Source: CAD feature listing. Evaluate the final solid. Frame: model axes, mm. A direction names the side the tool comes from. Give positions to 0.01 mm unless a question says otherwise; leave off trailing zeros. Loops run counter-clockwise (first coordinate to the right, second up) from the corner with the lowest first, then second, coordinate; pieces in that order, holes last. Notation, with made-up numbers: M -5,12.5 L 2,12.5 A19 cw 2,22.5 Z; hole C -29,4 d4. An arc over 180 degrees is marked long. Put each result on its own line as item: value.
from build123d import *

# Parameters (mm, degrees)
SKETCH1_W           = 166
SKETCH1_H           = 96
BOSS_EXTRUDE1_DEPTH = 33
SKETCH2_W           = 150
SKETCH2_H           = 80
CUT_EXTRUDE1_DEPTH  = 30
BOSS_EXTRUDE2_DEPTH = 5
SKETCH5_W           = 75
SKETCH5_H           = 5
BOSS_EXTRUDE3_DEPTH = 5
LPATTERN1_COUNT     = 15
LPATTERN1_PITCH     = 10
CUT_EXTRUDE5_DEPTH  = 10
FILLET1_R           = 4
FILLET2_R           = 4
FILLET3_R           = 2
FILLET5_R           = 1
CHAMFER1_SIZE       = 0.5


with BuildPart() as part:
    # Sketch1 → Boss-Extrude1 (new body)
    with BuildSketch(Plane(origin=(0, 0, 0), x_dir=(1, 0, 0), z_dir=(0, 1, 0))):
        with Locations((18.075570249, -18.706715624)):
            Rectangle(SKETCH1_W, SKETCH1_H)
    extrude(amount=BOSS_EXTRUDE1_DEPTH)

    # Sketch2 → Cut-Extrude1 (cut)
    with BuildSketch(Plane(origin=(0, 33, 0), x_dir=(1, 0, 0), z_dir=(0, 1, 0))):
        with Locations((18.075570249, -18.706715624)):
            Rectangle(SKETCH2_W, SKETCH2_H)
    extrude(amount=-CUT_EXTRUDE1_DEPTH, mode=Mode.SUBTRACT)

    # Sketch4 → Boss-Extrude2 (add)
    with BuildSketch(Plane.ZY.offset(-93.075570249)):
        Polygon((53.706715624, 3), (-21.293284376, 8), (-21.293284376, 3), align=None)
    boss_extrude2 = extrude(amount=BOSS_EXTRUDE2_DEPTH)

    # Sketch5 → Boss-Extrude3 (add)
    with BuildSketch(Plane.ZY.offset(-88.075570249)):
        with Locations((16.206715624, 5.5)):
            Rectangle(SKETCH5_W, SKETCH5_H)
    boss_extrude3 = extrude(amount=BOSS_EXTRUDE3_DEPTH)

    # LPattern1: Boss-Extrude2, Boss-Extrude3 ×15
    with Locations(*[(-i * LPATTERN1_PITCH, 0, 0) for i in range(1, LPATTERN1_COUNT)]):
        add(boss_extrude2)
        add(boss_extrude3)

    # Sketch9 → Cut-Extrude5 (cut)
    with BuildSketch(Plane(origin=(0, 33, 0), x_dir=(1, 0, 0), z_dir=(0, 1, 0))):
        Polygon((-62.174429751, 26.543284376), (98.325570249, 26.543284376), (98.325570249, -58.706715624), (95.325570249, -58.706715624), (95.325570249, 23.543284376), (-59.174429751, 23.543284376), (-59.174429751, -58.706715624), (-62.174429751, -58.706715624), align=None)
    extrude(amount=-CUT_EXTRUDE5_DEPTH, mode=Mode.SUBTRACT)

    # Fillet1
    fillet1_edges = [part.edges().sort_by_distance(p)[0] for p in [
        (-64.924429751, 16.5, -29.293284376),
        (101.075570249, 16.5, -29.293284376),
        (101.075570249, 16.5, 66.706715624),
        (-64.924429751, 16.5, 66.706715624),
    ]]
    fillet(fillet1_edges, radius=FILLET1_R)

    # Fillet2
    fillet2_edges = [part.edges().sort_by_distance(p)[0] for p in [
        (-56.924429751, 18, 58.706715624),
        (93.075570249, 18, 58.706715624),
        (93.075570249, 20.5, -21.293284376),
        (-56.924429751, 20.5, -21.293284376),
    ]]
    fillet(fillet2_edges, radius=FILLET2_R)

    # Fillet3
    fillet3_edges = [part.edges().sort_by_distance(p)[0] for p in [
        (75.575570249, 8, 53.706715624),
        (65.575570249, 8, 53.706715624),
        (55.575570249, 8, 53.706715624),
        (45.575570249, 8, 53.706715624),
        (35.575570249, 8, 53.706715624),
        (25.575570249, 8, 53.706715624),
        (15.575570249, 8, 53.706715624),
        (5.575570249, 8, 53.706715624),
        (-4.424429751, 8, 53.706715624),
        (-14.424429751, 8, 53.706715624),
        (-24.424429751, 8, 53.706715624),
        (-34.424429751, 8, 53.706715624),
        (-44.424429751, 8, 53.706715624),
        (-54.424429751, 8, 53.706715624),
        (85.575570249, 8, 53.706715624),
    ]]
    fillet(fillet3_edges, radius=FILLET3_R)

    # Fillet5
    fillet5_edges = [part.edges().sort_by_distance(p)[0] for p in [
        (-64.924429751, 33, 18.706715624),
        (18.075570249, 33, -29.293284376),
        (18.075570249, 33, 66.706715624),
        (101.075570249, 33, 18.706715624),
        (-63.752856875, 33, 65.535142749),
        (99.903997374, 33, 65.535142749),
        (99.903997374, 33, -28.1217115),
        (-63.752856875, 33, -28.1217115),
        (93.075570249, 33, 18.706715624),
        (18.075570249, 33, 58.706715624),
        (18.075570249, 33, -21.293284376),
        (-56.924429751, 33, 18.706715624),
        (91.903997374, 33, 57.535142749),
        (91.903997374, 33, -20.1217115),
        (-55.752856875, 33, -20.1217115),
        (-55.752856875, 33, 57.535142749),
    ]]
    fillet(fillet5_edges, radius=FILLET5_R)

    # Chamfer1
    chamfer1_edges = [part.edges().sort_by_distance(p)[0] for p in [
        (-62.174429751, 33, 16.081715624),
        (-60.674429751, 33, 58.706715624),
        (-59.174429751, 33, 17.581715624),
        (18.075570249, 33, -23.543284376),
        (95.325570249, 33, 17.581715624),
        (96.825570249, 33, 58.706715624),
        (98.325570249, 33, 16.081715624),
        (18.075570249, 33, -26.543284376),
    ]]
    chamfer(chamfer1_edges, length=CHAMFER1_SIZE)


solid = part.part
1. Access query for faces 1 (the flat face through (3.076, 7, 32)), 2 (the cylindrical face through (99.87, 16.22, 65.57)). Directions: +Z, -Z, +X, -X, +Y, -Y. A direction counts if a zero-diameter tool reaches every point of the face in a straight line with its end or side. Return the directions, or none.
Found:
face 1: +Y
face 2: +Z, +X, +Y, -Y
2. Section query A-A (y = 14). Output: boundary loops of the cut face in (x, z), plus the area to 3 significant figures.
Found:
outline: M -64.92,-25.29 A4 ccw -60.92,-29.29 L 97.08,-29.29 A4 ccw 101.08,-25.29 L 101.08,62.71 A4 ccw 97.08,66.71 L -60.92,66.71 A4 ccw -64.92,62.71 Z; hole M -56.92,-17.29 A4 ccw -52.92,-21.29 L 89.08,-21.29 A4 ccw 93.08,-17.29 L 93.08,54.71 A4 ccw 89.08,58.71 L -52.92,58.71 A4 ccw -56.92,54.71 Z
area: 3,940 mm^2
3. Section query B-B (x = 56). Output: boundary loops of the cut face in (y, z).
Found:
outline: M 0,-29.29 L 32,-29.29 A1 ccw 33,-28.29 L 33,-27.04 L 32.5,-26.54 L 23,-26.54 L 23,-23.54 L 32.5,-23.54 L 33,-23.04 L 33,-22.29 A1 ccw 32,-21.29 L 8,-21.29 L 8,51.71 A2 ccw 6,53.71 L 3,53.71 L 3,58.71 L 32,58.71 A1 ccw 33,59.71 L 33,65.71 A1 ccw 32,66.71 L 0,66.71 Z
4. Contact query for a flat-ended pin moving along its axis: P1, Ø5.5, axis at x = 66.5, z = 7, coming from the +Y side. Output: stop coordinate, or through.
Found:
P1: y = 8
5. Draft query along X for faces 3 (the flat face through (17, 16, -29.293)), 4 (the flat face through (10.611, 5.465, 16.732)), 5 (the cylindrical face through (99.873, 16.224, -28.153)). Return one class per face: pulls with the +X half, pulls with the -X half, needs draft (parallel to the pull), parting line crosses it, or undercut.
Found:
face 3: needs draft
face 4: undercut
face 5: pulls with the +X half
6. Material intervals for line 1 (Z direction, x = -16, y = 23.5); line 2 (X direction, y = 28, z = 18.5); line 3 (Z direction, x = -43, y = 5), sorted ascending. Write a range as from..to.
Found:
line 1: -29.29..-26.54, -23.54..-21.29, 58.71..66.71
line 2: -64.92..-62.17, -59.17..-56.92, 93.08..95.33, 98.33..101.08
line 3: -29.29..53.71, 58.71..66.71
